from build123d import *

# Parameters (mm, degrees)
EXTRUDE_1_DEPTH     = 1.5
SKETCH_2_R          = 0.45
SKETCH_2_R_2        = 1
SKETCH_2_R_3        = 0.4
SKETCH_2_R_4        = 0.7
CUT_EXTRUDE_1_DEPTH = 2.5


with BuildPart() as part:
    # Эскиз1 → Бобышка-Вытянуть1 (new body)
    with BuildSketch(Plane.XY):
        with BuildLine():
            Line((21, 12.5), (21, 7.481951683))
            ThreePointArc((21, 7.481951683), (30, 5.75), (39, 7.481951683))
            Line((39, 7.481951683), (39, 12.5))
            ThreePointArc((39, 12.5), (39.657111376, 13.439376065), (40.764854783, 13.144202733))
            ThreePointArc((40.764854783, 13.144202733), (30, 50), (19.235145217, 13.144202733))
            ThreePointArc((19.235145217, 13.144202733), (20.342888624, 13.439376065), (21, 12.5))
        make_face()
    extrude(amount=EXTRUDE_1_DEPTH)

    # Эскиз2 → Вырез-Вытянуть1 (cut, through all)
    with BuildSketch(Plane.XY.offset(1.5)):
        with Locations((34, 16)):
            Circle(SKETCH_2_R)
        with Locations((30, 44)):
            Circle(SKETCH_2_R_2)
        with Locations((13.5, 35)):
            Circle(SKETCH_2_R_3)
        with Locations((13.5, 25)):
            Circle(SKETCH_2_R_3)
        with Locations((18, 37)):
            Circle(SKETCH_2_R_4)
        with Locations((18, 23)):
            Circle(SKETCH_2_R_4)
        with BuildLine():
            Line((23.85, 35.5), (23.15, 35.5))
            ThreePointArc((23.15, 35.5), (22.15, 36.5), (23.15, 37.5))
            Line((23.15, 37.5), (23.85, 37.5))
            ThreePointArc((23.85, 37.5), (24.85, 36.5), (23.85, 35.5))
        make_face()
        with BuildLine():
            Line((36.85, 35.5), (36.15, 35.5))
            ThreePointArc((36.15, 35.5), (35.15, 36.5), (36.15, 37.5))
            Line((36.15, 37.5), (36.85, 37.5))
            ThreePointArc((36.85, 37.5), (37.85, 36.5), (36.85, 35.5))
        make_face()
        with BuildLine():
            Line((23.85, 22.5), (23.15, 22.5))
            ThreePointArc((23.15, 22.5), (22.15, 23.5), (23.15, 24.5))
            Line((23.15, 24.5), (23.85, 24.5))
            ThreePointArc((23.85, 24.5), (24.85, 23.5), (23.85, 22.5))
        make_face()
        with BuildLine():
            Line((36.85, 22.5), (36.15, 22.5))
            ThreePointArc((36.15, 22.5), (35.15, 23.5), (36.15, 24.5))
            Line((36.15, 24.5), (36.85, 24.5))
            ThreePointArc((36.85, 24.5), (37.85, 23.5), (36.85, 22.5))
        make_face()
        with BuildLine():
            Line((23.85, 8), (23.15, 8))
            ThreePointArc((23.15, 8), (22.15, 9), (23.15, 10))
            Line((23.15, 10), (23.85, 10))
            ThreePointArc((23.85, 10), (24.85, 9), (23.85, 8))
        make_face()
        with BuildLine():
            Line((36.85, 8), (36.15, 8))
            ThreePointArc((36.15, 8), (35.15, 9), (36.15, 10))
            Line((36.15, 10), (36.85, 10))
            ThreePointArc((36.85, 10), (37.85, 9), (36.85, 8))
        make_face()
    extrude(amount=-CUT_EXTRUDE_1_DEPTH, mode=Mode.SUBTRACT)


solid = part.part
Geometry: final body of the model. Coordinates: model frame, mm. A direction names the side the tool comes from. Coordinates: 2 decimals unless noted, no trailing zeros. Write each loop counter-clockwise with the first axis right and the second up, starting at its lowest first coordinate (ties: lowest second). Pieces come first, ordered by that corner, then holes. Notation, with made-up numbers: (64.5, 23.5) - (84.5, 23.5) arc R21 ccw to (84.5, 55.5) - close; hole circle Ø7 at (20, -32.5). An arc over 180 degrees is marked (long way). Return JSON: item names as keys, results as strings.
Item 1: Section query C-C (y = 37). Output: boundary loops of the cut face in (x, z) (3 decimals), and give its area (3 significant figures).
Completed:
{"outline": "(11.265, 0) - (17.3, 0) - (17.3, 1.5) - (11.265, 1.5) - close; (18.7, 0) - (22.284, 0) - (22.284, 1.5) - (18.7, 1.5) - close; (24.716, 0) - (35.284, 0) - (35.284, 1.5) - (24.716, 1.5) - close; (37.716, 0) - (48.735, 0) - (48.735, 1.5) - (37.716, 1.5) - close", "area": "46.8 mm2"}
Item 2: Section query A-A (y = 44). Output: boundary loops of the cut face in (x, z), and give its area (3 significant figures).
Completed:
{"outline": "(15.72, 0) - (29, 0) - (29, 1.5) - (15.72, 1.5) - close; (31, 0) - (44.28, 0) - (44.28, 1.5) - (31, 1.5) - close", "area": "39.8 mm2"}
Item 3: Section query D-D (z = 1.1). Count the separate pieces of the cut face and the enclosed holes in it, and give its area (3 significant figures).
Completed:
{"separate pieces": "1", "enclosed holes": "12", "area": "1,300 mm2"}
Item 4: Section query B-B (x = 30). Output: boundary loops of the cut face in (y, z), and give its area (3 significant figures).
Completed:
{"outline": "(5.75, 0) - (43, 0) - (43, 1.5) - (5.75, 1.5) - close; (45, 0) - (50, 0) - (50, 1.5) - (45, 1.5) - close", "area": "63.4 mm2"}
Item 5: Pin query (flat end, axial travel): pin 1 Ø0.8 at (x, z) = (36.5, 1) entering from +Y; pin 2 Ø0.8 at (x, z) = (23.5, 1) entering from -Y; pin 3 Ø2 at (x, y) = (45.5, 44.5) entering from -Z; pin 4 Ø1.6 at (x, y) = (18, 23) entering from -Z. Return the tip coordinate at first contact, or that it passes through.
Completed:
{"pin 1": "stops at y = 49.05", "pin 2": "stops at y = 6.53", "pin 3": "passes through", "pin 4": "stops at z = 0"}
Item 6: Reachability of faces 1 (the face through (30, 28, 0)), 2 (the face through (21, 10, 1)), 3 (the face through (24.85, 23.52, 0.76)) from +Z, -Z, +X, -X, +Y, -Y: full face, straight path, thin tool, end or side. Return the list, or none.
Completed:
{"face 1": "-Z, +X, -X, +Y, -Y", "face 2": "+Z, -Z, -X, -Y", "face 3": "+Z, -Z"}
Item 7: Line query: L1, parallel to Y at x = 18, z = 1.1; L2, parallel to X at y = 29.5, z = 0.1; L3, parallel to X at y = 41, z = 0.3. Output: solid intervals per line, ascending.
Completed:
{"L1": "y = 14 to 22.3, 23.7 to 36.3, 37.7 to 46", "L2": "x = 10.01 to 49.99", "L3": "x = 13.3 to 46.7"}
Item 8: Pull-direction query (Y, two-part tool) for faces 4 (the face through (30.72, 49.987, 0.74)), 5 (the face through (37.85, 9.02, 0.76)), 6 (the face through (20.327, 13.445, 0.74)); classes: +Y half, -Y half, draft (parallel to the pull), parting line (faces both ways), or undercut.
Completed:
{"face 4": "parting line", "face 5": "undercut", "face 6": "-Y half"}
